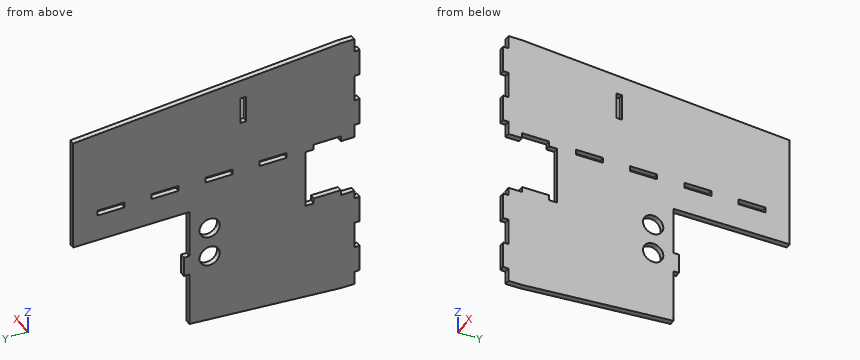
from build123d import *

# Parameters (mm, degrees)
SKICA1_W                = 20
SKICA1_H                = 4
SKICA1_W_2              = 4
SKICA1_H_2              = 20
SKICA1_R                = 7.5
P_IDAT_VYSUNUT_M1_DEPTH = 4


with BuildPart() as part:
    # Skica1 → Přidat vysunutím1 (new body)
    with BuildSketch(Plane(origin=(0, 0, 0), x_dir=(0, 0, -1), z_dir=(1, 0, 0))):
        Polygon((-20, 40), (24, 40), (24, 34), (20, 34), (20, 14), (24, 14), (24, 4), (30, 4), (30, 0), (50, 0), (50, 4), (70, 4), (70, 0), (90, 0), (90, 4), (100, 4), (100, 14), (91.515151515, 126), (51, 126), (51, 130), (36, 130), (36, 126), (0, 126), (0, 212), (-85, 212), (-100, 14), (-100, 4), (-90, 4), (-90, 0), (-70, 0), (-70, 4), (-50, 4), (-50, 0), (-30, 0), (-30, 4), (-20, 4), (-20, 14), (-24, 14), (-24, 34), (-20, 34), align=None)
        with Locations((-70, 86)):
            Rectangle(SKICA1_W, SKICA1_H, mode=Mode.SUBTRACT)
        with Locations((-22, 64)):
            Rectangle(SKICA1_W_2, SKICA1_H_2, mode=Mode.SUBTRACT)
        with Locations((-22, 104)):
            Rectangle(SKICA1_W_2, SKICA1_H_2, mode=Mode.SUBTRACT)
        with Locations((-22, 144)):
            Rectangle(SKICA1_W_2, SKICA1_H_2, mode=Mode.SUBTRACT)
        with Locations((-22, 184)):
            Rectangle(SKICA1_W_2, SKICA1_H_2, mode=Mode.SUBTRACT)
        with Locations((40.95225545, 111)):
            Circle(SKICA1_R, mode=Mode.SUBTRACT)
        with Locations((18.09225545, 111)):
            Circle(SKICA1_R, mode=Mode.SUBTRACT)
    extrude(amount=P_IDAT_VYSUNUT_M1_DEPTH)


solid = part.part
Read the model definition and answer for the solid it produces. Units are mm, in the model's axes. Round coordinates to 2 decimals unless told otherwise and drop trailing zeros. Order: outer loops, then holes, each group sorted by start corner. A loop starts at its lowest first (then second) coordinate and runs counter-clockwise, first axis right, second up. Notation, with made-up numbers: (67.5, -3.75) - (116.5, -3.75) arc R8 ccw to (116.5, 10.25) - close; hole circle Ø11 at (7, 43). An arc over 180 degrees is marked (long way). Use one line per item in the form item = value. Start each with the question number.
(1) Flat-ended cylindrical pins translate along their axes: pin 1 Ø2 at (x, y) = (2, 129.5) entering from -Z; pin 2 Ø2 at (x, z) = (2, 23) entering from -Y; pin 3 Ø2 at (x, y) = (3, 127.5) entering from +Z. Find the tip coordinate at first contact, or state that the pin passes through.
(2) Find the intervals of material crossed by line 1 along Y through (x, z) = (3.8, 74.5); line 2 along Z through (x, y) = (0.9, 114.5); line 3 along Y through (x, z) = (0.65, -74), in increasing order. Write a range as from..to.
(3) The part is cut by section A-A (z = -38.5). Give the vertices of the cut face in (x, y), then the cut area to 3 significant figures.
(4) The part is cut by section B-B (y = 25). Give the vertices of the cut face in (x, z), then the cut area to 3 significant figures.
(5) The part is cut by section D-D (x = 1.4). Count the separate pieces of the cut face and the enclosed holes in it, then the cut area to 3 significant figures.
(6) The part is cut by section C-C (y = 111). Give the vertices of the cut face in (x, z).
Checked values:
q1.pin_1 = -51
q1.pin_2 = 4
q1.pin_3 = 91.48
q2.line_1 = 0..84, 88..212
q2.line_2 = -92.39..-47.59, -34.32..-24.73, -11.46..92.39
q2.line_3 = 0..126
q3.outline = (0, 0) - (4, 0) - (4, 103.91) - (0, 103.91) - close; (0, 118.09) - (4, 118.09) - (4, 130) - (0, 130) - close
q3.area = 463 mm^2
q4.outline = (0, -99.17) - (4, -99.17) - (4, -20) - (0, -20) - close; (0, 24) - (4, 24) - (4, 99.17) - (0, 99.17) - close
q4.area = 617 mm^2
q5.separate_pieces = 1
q5.enclosed_holes = 7
q5.area = 29,100 mm^2
q6.outline = (0, -92.65) - (4, -92.65) - (4, -48.45) - (0, -48.45) - close; (0, -33.45) - (4, -33.45) - (4, -25.59) - (0, -25.59) - close; (0, -10.59) - (4, -10.59) - (4, 20) - (0, 20) - close; (0, 24) - (4, 24) - (4, 92.65) - (0, 92.65) - close
